Here's how the part is built. I have some questions about the finished solid (model axes, mm). A direction names the side the tool comes from. Give positions to 0.01 mm unless a question says otherwise; leave off trailing zeros. Loops run counter-clockwise (first coordinate to the right, second up) from the corner with the lowest first, then second, coordinate; pieces in that order, holes last. Notation, with made-up numbers: (69.5, -29) - (90.5, -29) arc R21 cw to (90.5, -16) - close; hole circle Ø5 at (-24.75, 8). An arc over 180 degrees is marked (long way). Use a Markdown table: item, result.
from build123d import *

# Parameters (mm, degrees)
SKETCH1_R           = 2.1
BOSS_EXTRUDE1_DEPTH = 5.08
FILLET1_R           = 2.54
FILLET2_R           = 10.16


with BuildPart() as part:
    # Sketch1 → Boss-Extrude1 (new body)
    with BuildSketch(Plane(origin=(0, 0, 0), x_dir=(1, 0, 0), z_dir=(0, 1, 0))):
        with BuildLine():
            ThreePointArc((0, 12.7), (-12.7, 0), (0, -12.7))
            Line((0, -12.7), (19.05, -12.7))
            Line((19.05, -12.7), (19.05, -38.1))
            Line((19.05, -38.1), (35.56, -38.1))
            Line((35.56, -38.1), (63.5, -38.1))
            Line((63.5, -38.1), (63.5, -12.7))
            Line((63.5, -12.7), (44.45, -12.7))
            Line((44.45, -12.7), (44.45, 12.7))
            Line((44.45, 12.7), (22.225, 12.7))
            Line((22.225, 12.7), (0, 12.7))
        make_face()
        with Locations((36.83, -25.4)):
            Circle(SKETCH1_R, mode=Mode.SUBTRACT)
        with Locations((48.26, -25.4)):
            Circle(SKETCH1_R, mode=Mode.SUBTRACT)
        Circle(SKETCH1_R, mode=Mode.SUBTRACT)
        with Locations((19.05, 0)):
            Circle(SKETCH1_R, mode=Mode.SUBTRACT)
        with Locations((30.48, 0)):
            Circle(SKETCH1_R, mode=Mode.SUBTRACT)
    extrude(amount=BOSS_EXTRUDE1_DEPTH)

    # Fillet1
    fillet1_edges = [part.edges().sort_by_distance(p)[0] for p in [
        (44.45, 2.54, 12.7),
        (19.05, 2.54, 12.7),
    ]]
    fillet(fillet1_edges, radius=FILLET1_R)

    # Fillet2
    fillet2_edges = [part.edges().sort_by_distance(p)[0] for p in [
        (44.45, 2.54, -12.7),
        (63.5, 2.54, 12.7),
        (63.5, 2.54, 38.1),
        (19.05, 2.54, 38.1),
    ]]
    fillet(fillet2_edges, radius=FILLET2_R)


solid = part.part
(1) We'd pull the mould along X, two halves only. Please class faces 1 (the face through (21.947, 2.576, 35.045)), 2 (the face through (44.45, 3, 4)), 3 (the face through (16.95, 2.5, -0.09)): pulls with the +X half, pulls with the -X half, needs draft (parallel to the pull), parting line crosses it, or undercut.
A:
| item | result |
|---|---|
| face 1 | pulls with the -X half |
| face 2 | pulls with the +X half |
| face 3 | undercut |
(2) On a 3-axis mill with a long thin cutter (end or side, diameter ignored), from which of +Z, -Z, +X, -X, +Y, -Y can I reach the whole of each face in a straight line? I mean faces 4 (the face through (8, 3, 12.7)), 5 (the face through (25, 5.08, 12)), 6 (the face through (50, 3, 12.7)). Say none if no direction works.
A:
| item | result |
|---|---|
| face 4 | +Z, -X, +Y, -Y |
| face 5 | +Z, -Z, +X, -X, +Y |
| face 6 | -Z, +X, +Y, -Y |
(3) If I drill on line 1 (X direction, y = 1.65, z = 25.4); line 2 (Z direction, x = 30.48, y = 1.5); line 3 (Z direction, x = 0, y = 1.1), over which ranges is the centre line in solid material (lowest first)?
A:
| item | result |
|---|---|
| line 1 | 19.05 to 34.73, 38.93 to 46.16, 50.36 to 63.5 |
| line 2 | -12.7 to -2.1, 2.1 to 38.1 |
| line 3 | -12.7 to -2.1, 2.1 to 12.7 |
(4) Suppose I cut it at C-C on z = 0. Write out the boundary of the cut face in (x, y), plus the area to 3 significant figures.
A:
| item | result |
|---|---|
| outline | (-12.7, 0) - (-2.1, 0) - (-2.1, 5.08) - (-12.7, 5.08) - close; (2.1, 0) - (16.95, 0) - (16.95, 5.08) - (2.1, 5.08) - close; (21.15, 0) - (28.38, 0) - (28.38, 5.08) - (21.15, 5.08) - close; (32.58, 0) - (44.45, 0) - (44.45, 5.08) - (32.58, 5.08) - close |
| area | 226 mm2 |
(5) Suppose I cut it at B-B on y = 0.85. Write out the boundary of the cut face in (x, z).
A:
| item | result |
|---|---|
| outline | (0, -12.7) - (34.29, -12.7) arc R10.16 ccw to (44.45, -2.54) - (44.45, 10.16) arc R2.54 cw to (46.99, 12.7) - (53.34, 12.7) arc R10.16 ccw to (63.5, 22.86) - (63.5, 27.94) arc R10.16 ccw to (53.34, 38.1) - (29.21, 38.1) arc R10.16 ccw to (19.05, 27.94) - (19.05, 15.24) arc R2.54 cw to (16.51, 12.7) - (0, 12.7) arc R12.7 ccw to start; hole circle Ø4.2 at (0, 0); hole circle Ø4.2 at (19.05, 0); hole circle Ø4.2 at (30.48, 0); hole circle Ø4.2 at (36.83, 25.4); hole circle Ø4.2 at (48.26, 25.4) |
(6) Suppose I cut it at D-D on z = 30.5. Write out the boundary of the cut face in (x, y).
A:
| item | result |
|---|---|
| outline | (19.38, 0) - (63.17, 0) - (63.17, 5.08) - (19.38, 5.08) - close |
(7) Will these pins go through, and if not, where does the flat tip stop? pin 1 (8 mm diameter, centred on x = 17.5, z = 29, fed in from -Y); pin 2 (1 mm diameter, centred on y = 2.5, z = 30, fed in from +X); pin 3 (2 mm diameter, centred on x = 46, y = 2.5, fed in from -Z); pin 4 (2.5 mm diameter, centred on x = 48.5, y = 3.5, fed in from -Z).
A:
| item | result |
|---|---|
| pin 1 | y = 0 |
| pin 2 | x = 63.38 |
| pin 3 | z = 11.74 |
| pin 4 | z = 12.7 |
(8) Suppose I cut it at A-A on x = 48.26. Write out the boundary of the cut face in (y, z).
A:
| item | result |
|---|---|
| outline | (0, 12.7) - (5.08, 12.7) - (5.08, 23.3) - (0, 23.3) - close; (0, 27.5) - (5.08, 27.5) - (5.08, 38.1) - (0, 38.1) - close |
